Autodesk Inventor part; units mm, degrees
ref_plane "YZ Plane" through (0, 0, 0) normal (1, 0, 0) x (0, 1, 0)
ref_plane "XZ Plane" through (0, 0, 0) normal (0, 1, 0) x (-1, 0, 0)
ref_plane "XY Plane" through (0, 0, 0) normal (0, 0, 1) x (1, 0, 0)
sketch "スケッチ1" plane through (0, 0, 0) normal (1, 0, 0) x (0, 1, 0)
  circle A0 centre (0, 0) radius 10
  circle A1 centre (0, -10) radius 1.35
  circle A2 centre (8.6603, 5) radius 1.35
  circle A3 centre (-8.6603, 5) radius 1.35
  circle A4 centre (0, 0) radius 5
  line L0 (0, 0) -> (0, 50)
  circle A5 centre (0, 50) radius 22.5
  circle A6 centre (0, 0) radius 14
  line L1 (-14, 0) -> (-22.5, 50)
  line L2 (14, 0) -> (22.5, 50)
  line L3 (0, -14) -> (-11.62, -14)
  line L4 (-11.62, -14) -> (-14, 0)
  line L5 (0, -14) -> (11.62, -14)
  line L6 (11.62, -14) -> (14, 0)
  line L7 (0, 20) -> (-17.4, 20)
  line L8 (0, 20) -> (17.4, 20)
  dimension "d0" = 20
  dimension "d1" = 2.7
  dimension "d4" = 360
  dimension "d6" = 10
  dimension "d7" = 50
  dimension "d8" = 45
  dimension "d9" = 28
extrude "押し出し1" add sketch "スケッチ1" along normal blind 4 contours A0 A1 A3 A2 | A6 L6 L4 | A6 L1 L7 L0 | L0 L8 L2 A6 | L6 L5 A6 | A6 L3 L4
sketch "スケッチ2" plane through (0, -17.4, 20) normal (0, 0, 1) x (1, 0, 0)
  line L0 (0, 17.4) -> (30, 17.4)
  circle A0 centre (30, 17.4) radius 22.5
  circle A1 centre (30, 17.4) radius 18.5
  circle A2 centre (30, 17.4) radius 14.25
  circle A3 centre (48.5, 17.4) radius 1.35
  circle A4 centre (20.75, 33.4215) radius 1.35
  circle A5 centre (20.75, 1.3785) radius 1.35
  line L1 (0, 29.02) -> (0, 34.8)
  line L2 (0, 0) -> (0, 5.78)
  line L3 (0, 34.8) -> (0, 0)
  line L4 (4, 29.02) -> (4, 34.8)
  line L5 (4, 34.8) -> (7, 34.8)
  line L6 (7, 34.8) -> (30, 39.9)
  line L7 (4, 0) -> (4, 5.78)
  line L8 (4, 0) -> (7, 0)
  line L9 (7, 0) -> (30, -5.1)
  line L10 (4, 0) -> (0, 0)
  line L11 (0, 34.8) -> (4, 34.8)
  line L12 (0, 0) -> (0, 34.8)
  line L13 (0, 34.8) -> (4, 34.8)
  dimension "d14" = 37
  dimension "d12" = 30
  dimension "d13" = 45
  dimension "d15" = 28.5
  dimension "d16" = 2.7
  dimension "d19" = 360
  dimension "d21" = 3
  dimension "d22" = 3
extrude "押し出し2" add sketch "スケッチ2" along normal blind 4 contours L3 L1 L11 L5 L6 A0 L0 | L0 A0 L9 L8 L10 L2 L3 | A1 A4 A3 A5 | A0 L6 L9
fillet "フィレット1" radius 3 2 edges at (4, 0, 20) (0, 0, 24)
fillet "フィレット2" radius 3 2 edges at (2, -11.62, -14) (2, 11.62, -14)
sketch "スケッチ7" plane through (0, -17.4, 24) normal (0, 0, 1) x (1, 0, 0)
  circle A0 centre (30, 17.4) radius 14.25
  line L0 (30, 17.4) -> (182.95, 17.4)
  line L1 (30, 17.4) -> (182.95, 17.4) construction
  circle A1 centre (182.95, 17.4) radius 3.5
  circle A2 centre (182.95, 17.4) radius 10
  line L2 (182.95, 27.4) -> (50.1556, 27.4)
  arc A3 (30, -5.1) -> (30, 39.9) centre (30, 17.4) ccw
  line L3 (182.95, 27.4) -> (315.7444, 27.4) construction
  line L4 (182.95, 7.4) -> (50.1556, 7.4)
  point P0 (0, 17.4)
  dimension "d55" = 152.95
  dimension "d56" = 0
  dimension "d57" = 7
  dimension "d58" = 20
  dimension "d59" = 180
extrude "押し出し7" add sketch "スケッチ7" against normal blind 4 contours A3 L2 A2 L0 | L0 A2 L4 A3 | A2
sketch "スケッチ8" plane through (0, -17.4, 24) normal (0, 0, 1) x (1, 0, 0)
  circle A0 centre (20.75, 33.4215) radius 1.35
  circle A1 centre (20.75, 33.4215) radius 2.5
  circle A2 centre (48.5, 17.4) radius 1.35
  circle A3 centre (48.5, 17.4) radius 2.5
  circle A4 centre (20.75, 1.3785) radius 1.35
  circle A5 centre (20.75, 1.3785) radius 2.5
  point P0 (0, 17.4)
  dimension "d63" = 5
  dimension "d64" = 5
  dimension "d65" = 5
extrude "押し出し8" cut sketch "スケッチ8" against normal blind 2 contours A0 | A1 | A3 | A4 | A5
fillet "フィレット4" radius 2 1 edges at (50.1556, 10, 22)
sketch "スケッチ11" plane through (0, -17.4, 24) normal (0, 0, 1) x (1, 0, 0)
  line L0 (51.36, 27.4) -> (182.95, 27.4)
  line L1 (182.95, 27.4) -> (202.95, 27.4)
  arc A0 (182.95, 7.4) -> (182.95, 27.4) centre (182.95, 17.4) ccw
  line L2 (182.95, 7.4) -> (207.95, 7.4)
  line L3 (207.95, 13.4) -> (207.95, 22.4)
  line L4 (207.95, 7.4) -> (231.95, 7.4)
  line L5 (232.95, 8.4) -> (232.95, 26.4)
  line L6 (231.95, 27.4) -> (228.95, 27.4)
  line L7 (227.95, 26.4) -> (227.95, 13.4)
  line L8 (226.95, 12.4) -> (208.95, 12.4)
  arc A1 (232.95, 26.4) -> (231.95, 27.4) centre (231.95, 26.4) ccw
  arc A2 (228.95, 27.4) -> (227.95, 26.4) centre (228.95, 26.4) ccw
  arc A3 (231.95, 7.4) -> (232.95, 8.4) centre (231.95, 8.4) ccw
  arc A4 (226.95, 12.4) -> (227.95, 13.4) centre (226.95, 13.4) ccw
  arc A5 (207.95, 13.4) -> (208.95, 12.4) centre (208.95, 13.4) ccw
  arc A6 (207.95, 22.4) -> (202.95, 27.4) centre (202.95, 22.4) ccw
  point P0 (0, 17.4)
  point P1 (207.95, 27.4)
  point P2 (232.95, 7.4)
  point P3 (232.95, 27.4)
  point P4 (227.95, 27.4)
  point P5 (227.95, 12.4)
  dimension "d83" = 25
  dimension "d84" = 25
  dimension "d85" = 20
  dimension "d86" = 5
  dimension "d87" = 15
  dimension "d88" = 1
  dimension "d89" = 5
extrude "押し出し11" add sketch "スケッチ11" against normal blind 4
properties part number "motor_holder_8-3" material "ABS プラスチック"
Can you work these out from the model? Positions are in its coordinate system, mm. A direction names the side the tool comes from. Coordinates: 2 decimals unless noted, no trailing zeros. Loops run counter-clockwise (first coordinate to the right, second up) from the corner with the lowest first, then second, coordinate; pieces in that order, holes last. Notation, with made-up numbers: (-30.5, 17.5) - (23.5, 17.5) arc R22 cw to (23.5, 33.5) - close; hole circle Ø6 at (46, -30). An arc over 180 degrees is marked (long way). Answer as CSV lines item,"result". Start each with the question number.
1) Which directions (+Z, -Z, +X, -X, +Y, -Y) give clear straight access to the entire face, cutting with the end or side of a thin tool? Please do faces 1 (the flat face through (22, -17, 22)), 2 (the flat face through (4, -0.2, 5.2)), 3 (the flat face through (207.95, 0, 22)).
2) Thinking about a two-plate mould opening in X: for faces 4 (the cylindrical face through (179.453, 0.154, 22.028)), 5 (the flat face through (2, 0, -14)), 6 (the flat face through (18.339, 19.914, 21.972)), which applies, pulls with the +X half, pulls with the -X half, needs draft (parallel to the pull), parting line crosses it, or undercut?
3) Suppose I cut it at A-A (x = 182.95). Please give me the cut outline in (y, z), plus the area to 3 significant figures.
4) For pin 1 (5 mm diameter, centred on x = 145.5, y = -2.5, fed in from -Z); pin 2 (2 mm diameter, centred on y = 12.5, z = -2.5, fed in from +X); pin 3 (1.2 mm diameter, centred on x = 128, z = 22, fed in from +Y), each with a flat end and sliding along its axis, tell me the tip position at first contact or that it passes through.
5) I need wall thicknesses on line 1 (Z direction, x = 53, y = 2); line 2 (Y direction, x = 2, z = 0); line 3 (X direction, y = -4.5, z = 3). Which ranges of each line are inside material? Lowest first, please. Write a range as from..to.
6) Suppose I cut it at B-B (z = 0). Please give me the cut outline in (x, y).
Check result:
1,face 1,"+Z"
1,face 2,"-Z, +X, +Y, -Y"
1,face 3,"+Z, -Z, +Y"
2,face 4,"undercut"
2,face 5,"needs draft"
2,face 6,"pulls with the -X half"
3,outline,"(-10, 20) - (-3.5, 20) - (-3.5, 24) - (-10, 24) - close; (3.5, 20) - (10, 20) - (10, 24) - (3.5, 24) - close"
3,area,"52.0 mm²"
4,pin 1,"stops at z = 20"
4,pin 2,"stops at x = 4"
4,pin 3,"stops at y = 10"
5,line 1,"z = 20..24"
5,line 2,"y = -14..-5, 5..14"
5,line 3,"x = 0..4"
6,outline,"(0, -14) - (4, -14) - (4, -5) - (0, -5) - close; (0, 5) - (4, 5) - (4, 14) - (0, 14) - close"
